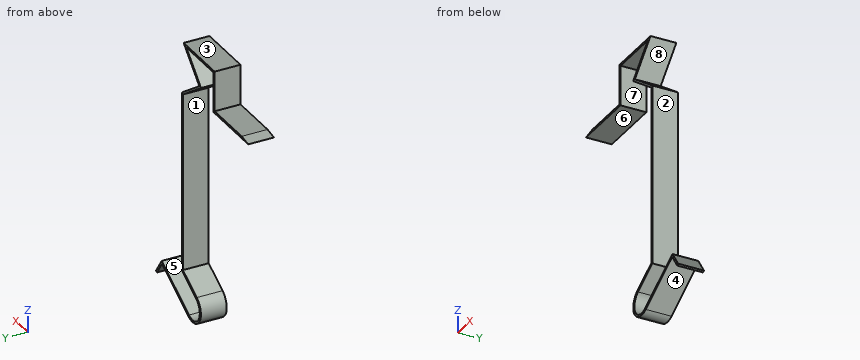
from build123d import *

# Parameters (mm, degrees)
EXTRUDE_1_DEPTH = 2.5


with BuildPart() as part:
    # 草图1 → 凸台-拉伸1 (new body)
    with BuildSketch(Plane(origin=(0, 0, 0), x_dir=(1, 0, 0), z_dir=(0, 1, 0))):
        with BuildLine():
            Line((-10.934737319, 12.934852592), (-4.684737319, 12.934852592))
            Line((-4.684737319, 12.934852592), (-4.684737319, 9.034852592))
            Line((-4.684737319, 9.034852592), (0.232419968, 9.034852592))
            Line((0.232419968, 9.034852592), (-2.42312521, 11.69039777))
            Line((-2.42312521, 11.69039777), (0.853482967, 13.984703515))
            Line((0.853482967, 13.984703515), (0.853482967, 31.265120051))
            Line((0.853482967, 31.265120051), (-1.644593244, 32.707385024))
            ThreePointArc((-1.644593244, 32.707385024), (-2.19363135, 34.75642313), (-0.144593244, 35.305461236))
            Line((-0.144593244, 35.305461236), (4.618546477, 32.555461236))
            Line((4.618546477, 32.555461236), (5.538541961, 33.864509863))
            Line((5.538541961, 33.864509863), (5.712435322, 33.764112484))
            Line((5.712435322, 33.764112484), (4.676983419, 32.290782544))
            Line((4.676983419, 32.290782544), (-0.244593244, 35.132256155))
            ThreePointArc((-0.244593244, 35.132256155), (-2.020426269, 34.65642313), (-1.544593244, 32.880590105))
            Line((-1.544593244, 32.880590105), (1.053482967, 31.380590105))
            Line((1.053482967, 31.380590105), (1.053482967, 13.880590105))
            Line((1.053482967, 13.880590105), (-2.113164444, 11.663279717))
            Line((-2.113164444, 11.663279717), (0.715262681, 8.834852592))
            Line((0.715262681, 8.834852592), (-4.884737319, 8.834852592))
            Line((-4.884737319, 8.834852592), (-4.884737319, 12.734852592))
            Line((-4.884737319, 12.734852592), (-9.767685017, 12.734852592))
            Line((-9.767685017, 12.734852592), (-10.934737319, 12.934852592))
        make_face()
    extrude(amount=EXTRUDE_1_DEPTH)


solid = part.part
Check sheet for the modelled part. Datum: model origin and axes. Units: mm. Face numbers are marked on the shaded views. A direction names the side the tool comes from. Round coordinates to 2 decimals unless told otherwise and drop trailing zeros. Order: outer loops, then holes, each group sorted by start corner. A loop starts at its lowest first (then second) coordinate and runs counter-clockwise, first axis right, second up.
(1) Draft check along Z on the marked faces 1, 2, 3 and 4. Enter one of: pulls with the +Z half, pulls with the -Z half, needs draft (parallel to the pull), parting line crosses it, or undercut.
(2) Access from +Z, -Z, +X, -X, +Y, -Y to the whole of each face (thin tool, end or side, straight path). Record for the marked faces 5, 6, 7 and 8.
(3) Cross-section at B-B, the plane y = 0.85. Enter the section's corners in (x, z).
(4) Cross-section at C-C, the plane z = -33.25. Enter the section's corners in (x, y).
(5) Cross-section at A-A, the plane z = -11. Enter the section's corners in (x, y), and give its area (3 significant figures).
(6) Scan lines: probe 1 along Z at (x, y) = (-1, 1.4); probe 2 along X at (y, z) = (1.8, -27.25); probe 3 along Z at (x, y) = (-9.5, 0.2). Record each from-to range of solid material in increasing order.
(7) Go/stop test with flat-tipped pins: P1, Ø1.2, axis at y = 1.5, z = -11.5, coming from the -X side; P2, Ø1.2, axis at y = 1, z = -23, coming from the +X side; P3, Ø0.8, axis at x = -7, y = 1, coming from the +Z side. Record where each tip stops, or that it passes through.
(8) Cross-section at D-D, the plane x = -7. Enter the section's corners in (y, z).
Check sheet entries:
1. face 1: undercut
1. face 2: needs draft
1. face 3: pulls with the +Z half
1. face 4: pulls with the -Z half
2. face 5: +Y, -Y
2. face 6: -Z, -X, +Y, -Y
2. face 7: -Z, +Y, -Y
2. face 8: +X, +Y, -Y
3. outline: (-10.93, -12.93) - (-4.68, -12.93) - (-4.68, -9.03) - (0.23, -9.03) - (-2.42, -11.69) - (0.85, -13.98) - (0.85, -31.27) - (-1.64, -32.71) arc R1.5 ccw to (-0.14, -35.31) - (4.62, -32.56) - (5.54, -33.86) - (5.71, -33.76) - (4.68, -32.29) - (-0.24, -35.13) arc R1.3 cw to (-1.54, -32.88) - (1.05, -31.38) - (1.05, -13.88) - (-2.11, -11.66) - (0.72, -8.83) - (-4.88, -8.83) - (-4.88, -12.73) - (-9.77, -12.73) - close
4. outline: (-2.19, 0) - (-1.95, 0) - (-1.95, 2.5) - (-2.19, 2.5) - close; (3.02, 0) - (3.42, 0) - (3.42, 2.5) - (3.02, 2.5) - close; (5.11, 0) - (5.35, 0) - (5.35, 2.5) - (5.11, 2.5) - close
5. outline: (-4.88, 0) - (-4.68, 0) - (-4.68, 2.5) - (-4.88, 2.5) - close; (-1.73, 0) - (-1.45, 0) - (-1.45, 2.5) - (-1.73, 2.5) - close
5. area: 1.21 mm2
6. probe 1: z = -35.5 to -35.3, -32.57 to -32.34, -12.69 to -12.44, -10.55 to -10.27, -9.03 to -8.83
6. probe 2: x = 0.85 to 1.05
6. probe 3: z = -12.93 to -12.73
7. P1: stops at x = -4.88
7. P2: stops at x = 1.05
7. P3: stops at z = -12.73
8. outline: (0, -12.93) - (2.5, -12.93) - (2.5, -12.73) - (0, -12.73) - close
